```python
from build123d import *

# Parameters (mm, degrees)
BOSS_EXTRUDE1_DEPTH = 8
SKETCH2_W           = 23.137445614
SKETCH2_H           = 10.306738945
BOSS_EXTRUDE2_DEPTH = 8


with BuildPart() as part:
    # Sketch1 → Boss-Extrude1 (new body)
    with BuildSketch(Plane(origin=(0, 0, 0), x_dir=(1, 0, 0), z_dir=(0, 1, 0))):
        with BuildLine():
            Line((11.568722807, -17.464704369), (11.568722807, 17.464704369))
            Line((11.568722807, 17.464704369), (0, 17.464704369))
            Line((0, 17.464704369), (0, -2.002357687))
            ThreePointArc((0, -2.002357687), (4.242640687, -3.759717), (6, -8.002357687))
            ThreePointArc((6, -8.002357687), (4.242640687, -12.244998375), (0, -14.002357687))
            Line((0, -14.002357687), (0, -17.464704369))
            Line((0, -17.464704369), (11.568722807, -17.464704369))
        make_face()
        with BuildLine():
            Line((0, -2.002357687), (0, 17.464704369))
            Line((0, 17.464704369), (-11.568722807, 17.464704369))
            Line((-11.568722807, 17.464704369), (-11.568722807, -17.464704369))
            Line((-11.568722807, -17.464704369), (0, -17.464704369))
            Line((0, -17.464704369), (0, -14.002357687))
            ThreePointArc((0, -14.002357687), (-6, -8.002357687), (0, -2.002357687))
        make_face()
    extrude(amount=BOSS_EXTRUDE1_DEPTH)

    # Sketch2 → Boss-Extrude2 (add)
    with BuildSketch(Plane.XZ):
        with Locations((0, -22.618073841)):
            Rectangle(SKETCH2_W, SKETCH2_H)
    extrude(amount=-BOSS_EXTRUDE2_DEPTH)


solid = part.part
```
Could you check a few things on this model? Use its own coordinates, in mm. Coordinates: 2 decimals unless noted, no trailing zeros. Order: outer loops, then holes, each group sorted by start corner. A loop starts at its lowest first (then second) coordinate and runs counter-clockwise, first axis right, second up. Notation, with made-up numbers: M -35,87 L 12,87 A4 ccw 12,94 Z; hole C -17.75,37.25 d5. An arc over 180 degrees is marked long. Use one line per item in the form item = value. Start each with the question number.
1. Suppose I cut it at A-A on z = 10. Write out the boundary of the cut face in (x, y), then the cut area to 3 significant figures.
2. Suppose I cut it at B-B on y = 1. Write out the boundary of the cut face in (x, z), then the cut area to 3 significant figures.
3. Please list where these lines run through material, in increasing order: line 1 (Z direction, x = -0.25, y = 5.75); line 2 (X direction, y = 3, z = 13.5); line 3 (X direction, y = 5.25, z = 13).
Geometry says:
q1.outline = M -11.57,0 L -5.66,0 L -5.66,8 L -11.57,8 Z; M 5.66,0 L 11.57,0 L 11.57,8 L 5.66,8 Z
q1.area = 94.6 mm^2
q2.outline = M -11.57,-27.77 L 11.57,-27.77 L 11.57,17.46 L -11.57,17.46 Z; hole C 0,8 d12
q2.area = 934 mm^2
q3.line_1 = -27.77 to 2.01, 14 to 17.46
q3.line_2 = -11.57 to -2.4, 2.4 to 11.57
q3.line_3 = -11.57 to -3.32, 3.32 to 11.57
